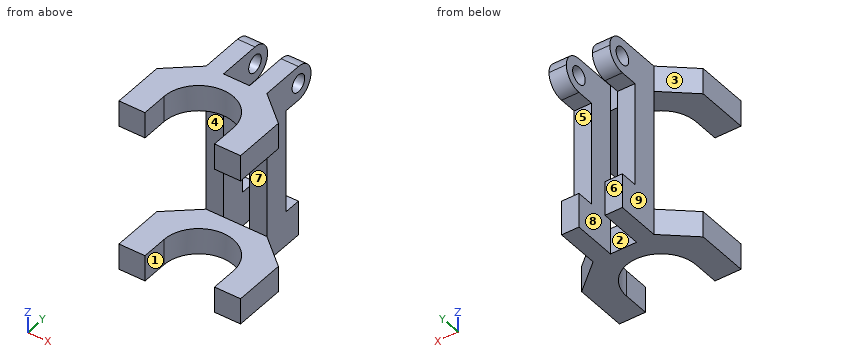
from build123d import *

# Parameters (mm, degrees)
BOSS_EXTRUDE1_DEPTH = 127
SKETCH3_W           = 88.9
SKETCH3_H           = 57.15
CUT_EXTRUDE1_DEPTH  = 166.222070257
SKETCH5_W           = 44.45
SKETCH5_H           = 44.45
BOSS_EXTRUDE2_DEPTH = 127
CUT_EXTRUDE2_DEPTH  = 176.775753803
FILLET1_R           = 12.7
SKETCH8_R           = 6.35
CUT_EXTRUDE3_DEPTH  = 176.775753803
SKETCH9_W           = 19.05
SKETCH9_H           = 44.45
CUT_EXTRUDE4_DEPTH  = 186.350397895


with BuildPart() as part:
    # Sketch2 → Boss-Extrude1 (new body)
    with BuildSketch(Plane.XY):
        with BuildLine():
            Line((0, 0), (19.05, 0))
            Line((19.05, 0), (19.05, 19.05))
            ThreePointArc((19.05, 19.05), (44.45, 44.45), (69.85, 19.05))
            Line((69.85, 19.05), (69.85, 0))
            Line((69.85, 0), (88.9, 0))
            Line((88.9, 0), (88.9, 38.1))
            Line((88.9, 38.1), (66.675, 57.15))
            Line((66.675, 57.15), (22.225, 57.15))
            Line((22.225, 57.15), (0, 38.1))
            Line((0, 38.1), (0, 0))
        make_face()
    extrude(amount=-BOSS_EXTRUDE1_DEPTH)

    # Sketch3 → Cut-Extrude1 (cut, through all)
    with BuildSketch(Plane(origin=(88.9, 0, 0), x_dir=(0, 0, -1), z_dir=(1, 0, 0))):
        with Locations((63.5, 28.575)):
            Rectangle(SKETCH3_W, SKETCH3_H)
    extrude(amount=-CUT_EXTRUDE1_DEPTH, mode=Mode.SUBTRACT)


with BuildPart() as cut_extrude1_piece_1:
    # of the separate pieces the step leaves, piece 1, a body of its own (cut_extrude1_pieces)
    add(part.part.solids().sort_by_distance((0, 0, 0))[0])



with BuildPart() as cut_extrude1_piece_2:
    # of the separate pieces the step leaves, piece 2, a body of its own (cut_extrude1_pieces)
    add(part.part.solids().sort_by_distance((19.05, 0, -107.95))[0])


with BuildPart() as cut_extrude1_piece_1_1:
    add(cut_extrude1_piece_1.part)

    add(cut_extrude1_piece_2.part)  # Boss-Extrude2 merges Cut-Extrude1 piece 2
    # Sketch5 → Boss-Extrude2 (add)
    with BuildSketch(Plane.XY):
        with Locations((44.45, 79.375)):
            Rectangle(SKETCH5_W, SKETCH5_H)
    extrude(amount=-BOSS_EXTRUDE2_DEPTH)

    # Sketch6 → Cut-Extrude2 (cut, through all)
    with BuildSketch(Plane(origin=(66.675, 0, 0), x_dir=(0, 0, -1), z_dir=(1, 0, 0))):
        Polygon((127, 88.9), (101.6, 88.9), (101.6, 76.2), (25.4, 76.2), (25.4, 101.6), (127, 101.6), align=None)
    extrude(amount=-CUT_EXTRUDE2_DEPTH, mode=Mode.SUBTRACT)

    # Fillet1
    fillet1_edges = [cut_extrude1_piece_1_1.edges().sort_by_distance(p)[0] for p in [
        (44.45, 101.6, -25.4),
        (44.45, 101.6, 0),
    ]]
    fillet(fillet1_edges, radius=FILLET1_R - 0.0001)  # a hair under: the kernel refuses the full size

    # Sketch8 → Cut-Extrude3 (cut, through all)
    with BuildSketch(Plane(origin=(66.675, 0, 0), x_dir=(0, 0, -1), z_dir=(1, 0, 0))):
        with Locations((12.7, 88.9)):
            Circle(SKETCH8_R)
    extrude(amount=-CUT_EXTRUDE3_DEPTH, mode=Mode.SUBTRACT)

    # Sketch9 → Cut-Extrude4 (cut, through all)
    with BuildSketch(Plane.XY):
        with Locations((44.45, 79.375)):
            Rectangle(SKETCH9_W, SKETCH9_H)
    extrude(amount=-CUT_EXTRUDE4_DEPTH, mode=Mode.SUBTRACT)


solid = cut_extrude1_piece_1_1.part
For this review, take the finished solid that the model builds, in its own axes (mm). Face numbers are marked on the shaded views. A direction names the side the tool comes from. Round coordinates to 2 decimals unless told otherwise and drop trailing zeros. Loops run counter-clockwise (first coordinate to the right, second up) from the corner with the lowest first, then second, coordinate; pieces in that order, holes last. Notation, with made-up numbers: (-5, 19.25) - (54, 19.25) arc R15 ccw to (54, 28.25) - close; hole circle Ø5 at (6.5, 72). An arc over 180 degrees is marked (long way). Answer as CSV lines item,"result".
(1) Mouldability with a two-part tool opening along X and no side actions: class the marked faces 1, 2, 3 and 4 as +X half, -X half, draft (parallel to the pull), parting line (faces both ways), or undercut.
Checked values:
face 1,"undercut"
face 2,"undercut"
face 3,"-X half"
face 4,"draft"
(2) Consider section A-A on z = -103.5. Give the boundary of the cut face in (x, y) (3 decimals).
Checked values:
outline,"(22.225, 57.15) - (34.925, 57.15) - (34.925, 88.9) - (22.225, 88.9) - close; (53.975, 57.15) - (66.675, 57.15) - (66.675, 88.9) - (53.975, 88.9) - close"
(3) Tool access review of the marked faces 5, 6, 7, 8 and 9: name each direction out of +Z, -Z, +X, -X, +Y, -Y from which nothing blocks a thin tool from reaching the whole face with its end or side.
Checked values:
face 5,"+X, -X, +Y"
face 6,"-Z, +X, -X, +Y"
face 7,"+X, -X, -Y"
face 8,"+Z, -Z, +Y"
face 9,"+Z, -Z, -X, +Y"
(4) Wall thickness on line 1 (Z direction, x = 15, y = 14); line 2 (Z direction, x = 30, y = 88); line 3 (X direction, y = 5.5, z = -120.5): over which ranges is each line inside the solid? List them lowest first.
Checked values:
line 1,"z = -127 to -107.95, -19.05 to 0"
line 2,"z = -127 to -101.6, -25.4 to -18.99, -6.41 to 0"
line 3,"x = 0 to 19.05, 69.85 to 88.9"
(5) Consider section D-D on y = 32.5. Give the boundary of the cut face in (x, z).
Checked values:
outline,"(0, -127) - (22.9, -127) - (22.9, -107.95) - (0, -107.95) - close; (0, -19.05) - (22.9, -19.05) - (22.9, 0) - (0, 0) - close; (66, -127) - (88.9, -127) - (88.9, -107.95) - (66, -107.95) - close; (66, -19.05) - (88.9, -19.05) - (88.9, 0) - (66, 0) - close"
(6) Insertion check: P1, Ø3, axis at x = 31.5, z = -62.5, coming from the +Y side; P2, Ø15, axis at x = 43, z = -13.5, coming from the +Y side; P3, Ø6.5, axis at x = 29, z = -44.5, coming from the -Y side; P4, Ø1, axis at y = 35.5, z = -106.5, coming from the -X side. Each pin has a flat end and moves straight along its axis. Give the tip position at first contact, or say it passes through.
Checked values:
P1,"stops at y = 76.2"
P2,"stops at y = 57.15"
P3,"stops at y = 57.15"
P4,"passes through"
(7) Consider section B-B on y = 52.5. Give the boundary of the cut face in (x, z), then the cut area to 3 significant figures.
Checked values:
outline,"(16.8, -127) - (72.1, -127) - (72.1, -107.95) - (16.8, -107.95) - close; (16.8, -19.05) - (72.1, -19.05) - (72.1, 0) - (16.8, 0) - close"
area,"2,110 mm2"
